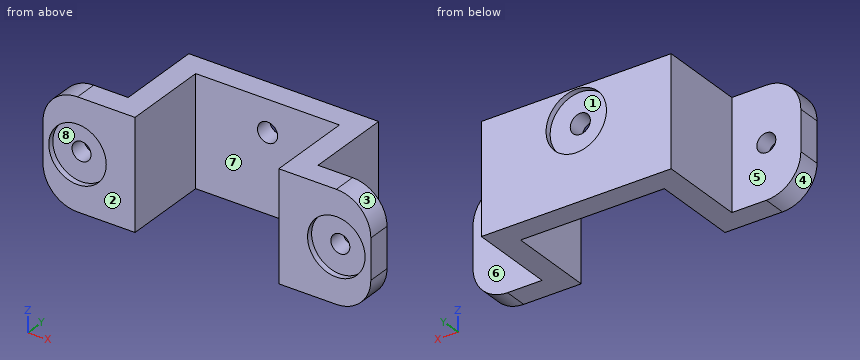
from build123d import *

# Parameters (mm, degrees)
RESSALTO_EXTRUS_O1_DEPTH   = 19
ESBO_O2_R                  = 1.75
ESBO_O2_R_2                = 1.65
CORTE_EXTRUS_O1_DEPTH      = 1
CORTE_EXTRUS_O1_DEPTH_BACK = 20
FILETE1_R                  = 6
ESBO_O3_R                  = 5
CORTE_EXTRUS_O2_DEPTH      = 1
ESBO_O4_R                  = 5.25
CORTE_EXTRUS_O3_DEPTH      = 1


with BuildPart() as part:
    # Esboço1 → Ressalto-extrusão1 (new body)
    with BuildSketch(Plane.XY):
        Polygon((12.5, 15), (-12.5, 15), (-12.5, 0), (-28.5, 0), (-28.5, 4), (-16.5, 4), (-16.5, 19), (16.5, 19), (16.5, 4), (28.5, 4), (28.5, 0), (12.5, 0), align=None)
    extrude(amount=RESSALTO_EXTRUS_O1_DEPTH)

    # Esboço2 → Corte-extrusão1 (cut, two sides)
    with BuildSketch(Plane(origin=(0, 19, 0), x_dir=(1, 0, 0), z_dir=(0, 1, 0))) as corte_extrus_o1_sk:
        with Locations((0, -13.5)):
            Circle(ESBO_O2_R)
        with Locations((-22.5, -9.5)):
            Circle(ESBO_O2_R_2)
        with Locations((22.5, -9.5)):
            Circle(ESBO_O2_R_2)
    extrude(amount=CORTE_EXTRUS_O1_DEPTH, mode=Mode.SUBTRACT)
    extrude(corte_extrus_o1_sk.sketch, amount=-CORTE_EXTRUS_O1_DEPTH_BACK, mode=Mode.SUBTRACT)

    # Filete1
    filete1_edges = [part.edges().sort_by_distance(p)[0] for p in [
        (28.5, 2, 0),
        (-28.5, 2, 0),
        (-28.5, 2, 19),
        (28.5, 2, 19),
    ]]
    fillet(filete1_edges, radius=FILETE1_R)

    # Esboço3 → Corte-extrusão2 (cut)
    with BuildSketch(Plane.XZ):
        with Locations((-22.5, 9.5)):
            Circle(ESBO_O3_R)
        with Locations((22.5, 9.5)):
            Circle(ESBO_O3_R)
    extrude(amount=-CORTE_EXTRUS_O2_DEPTH, mode=Mode.SUBTRACT)

    # Esboço4 → Corte-extrusão3 (cut)
    with BuildSketch(Plane(origin=(0, 19, 0), x_dir=(1, 0, 0), z_dir=(0, 1, 0))):
        with Locations((0, -13.5)):
            Circle(ESBO_O4_R)
    extrude(amount=-CORTE_EXTRUS_O3_DEPTH, mode=Mode.SUBTRACT)


solid = part.part
The listing builds one solid part. Answer for the finished solid, in the listing's coordinates (mm). Face numbers are marked on the shaded views. A direction names the side the tool comes from. Coordinates: 2 decimals unless noted, no trailing zeros. Loops run counter-clockwise (first coordinate to the right, second up) from the corner with the lowest first, then second, coordinate; pieces in that order, holes last. Notation, with made-up numbers: M 31.25,-9.75 L 78.25,-9.75 A24 cw 78.25,6.25 Z; hole C -29.5,42.5 d4. An arc over 180 degrees is marked long. Answer in a Markdown table with one row per item.
1) Find section B-B (y = 8.5). Determine the outline of the cut face in (x, z), then the cut area to 3 significant figures.
Answers below:
| item | result |
|---|---|
| outline | M -16.5,0 L -12.5,0 L -12.5,19 L -16.5,19 Z; M 12.5,0 L 16.5,0 L 16.5,19 L 12.5,19 Z |
| area | 152 mm^2 |
2) Determine the mould class of the marked faces 1, 2 and 3 for opening direction X: released by +X, released by -X, zero draft, split by the parting line, or undercut.
Answers below:
| item | result |
|---|---|
| face 1 | undercut |
| face 2 | zero draft |
| face 3 | released by +X |
3) Find section A-A (x = 0). Determine the outline of the cut face in (y, z), then the cut area to 3 significant figures.
Answers below:
| item | result |
|---|---|
| outline | M 15,0 L 19,0 L 19,8.25 L 18,8.25 L 18,11.75 L 15,11.75 Z; M 15,15.25 L 18,15.25 L 18,18.75 L 19,18.75 L 19,19 L 15,19 Z |
| area | 55.0 mm^2 |
4) Find the intervals of material crossed by probe 1 along X at (y, z) = (13.5, 1.75); probe 2 along X at (y, z) = (17.25, 13.5); probe 3 along Y at (x, z) = (5.5, 7), in increasing order.
Answers below:
| item | result |
|---|---|
| probe 1 | -16.5 to -12.5, 12.5 to 16.5 |
| probe 2 | -16.5 to -1.75, 1.75 to 16.5 |
| probe 3 | 15 to 19 |
5) Which of the six approach directions +Z, -Z, +X, -X, +Y, -Y give full straight-line access (tool end or side, diameter ignored) to the marked faces 4, 5, 6, 7 and 8?
Answers below:
| item | result |
|---|---|
| face 4 | -Z, -X, +Y, -Y |
| face 5 | +Z, -Z, -X, +Y |
| face 6 | +Z, -Z, +X, +Y |
| face 7 | +Z, -Z, -Y |
| face 8 | -Y |
6) Find section C-C (z = 9.5). Count the separate pieces of the cut face and the enclosed holes in it, then the cut area to 3 significant figures.
Answers below:
| item | result |
|---|---|
| separate pieces | 3 |
| enclosed holes | 0 |
| area | 301 mm^2 |
7) Find section D-D (x = -19). Determine the outline of the cut face in (y, z).
Answers below:
| item | result |
|---|---|
| outline | M 0,0 L 4,0 L 4,19 L 0,19 L 0,13.07 L 1,13.07 L 1,5.93 L 0,5.93 Z |
8) Given pin 1 (4.5 mm diameter, centred on x = 0, z = 13.5, fed in from -Y); pin 2 (3.5 mm diameter, centred on x = 24, z = 7.5, fed in from +Y); pin 3 (7.5 mm diameter, centred on y = 10, z = 7.5, fed in from +X), each flat-ended and moving along its own axis, determine where each tip first touches the part or whether it passes through.
Answers below:
| item | result |
|---|---|
| pin 1 | y = 15 |
| pin 2 | y = 4 |
| pin 3 | x = 16.5 |
